```python
from build123d import *

# Parameters (mm, degrees)
CUT_EXTRUDE1_DEPTH  = 3
BOSS_EXTRUDE1_START = 15
SKETCH12_R          = 2
BOSS_EXTRUDE1_DEPTH = 15


with BuildPart() as part:
    # Sketch2 → Revolve1 (revolve)
    with BuildSketch(Plane(origin=(0, 0, 0), x_dir=(0, 0, -1), z_dir=(1, 0, 0))):
        with BuildLine():
            Line((-7, 0), (-7, 3.3))
            Line((-7, 3.3), (-6.8, 3.5))
            Line((-6.8, 3.5), (-3.2, 3.5))
            Line((-3.2, 3.5), (-3, 3.3))
            Line((-3, 3.3), (-3, 2.2))
            ThreePointArc((-3, 2.2), (-2.941421356, 2.058578644), (-2.8, 2))
            Line((-2.8, 2), (6.545336663, 2))
            Line((6.545336663, 2), (7, 1.545336663))
            Line((7, 1.545336663), (7, 0))
            Line((7, 0), (-7, 0))
        make_face()
    revolve(axis=Axis((0, 0, -7), (0, 0, 1)))

    # Sketch3 → Cut-Extrude1 (cut)
    with BuildSketch(Plane.XY.offset(7)):
        Polygon((1.5, -0.866025404), (1.5, 0.866025404), (0, 1.732050808), (-1.5, 0.866025404), (-1.5, -0.866025404), (0, -1.732050808), align=None)
    extrude(amount=-CUT_EXTRUDE1_DEPTH, mode=Mode.SUBTRACT)

    # Cut-Extrude2 cone 1 section (through the dimple's axis) → Cut-Extrude2 (revolve, cut)
    with BuildSketch(Plane(origin=(0, 0, 7), x_dir=(0, -1, 0), z_dir=(1, 0, 0))):
        Polygon((0, 0), (1.875, 0), (0, 1.875), align=None)
    revolve(axis=Axis((0, 0, 7), (0, 0, -1)), mode=Mode.SUBTRACT)

    # Sketch12 → Boss-Extrude1 (add)
    with BuildSketch(Plane(origin=(0, 0, 3), x_dir=(-1, 0, 0), z_dir=(0, 0, -1)).offset(BOSS_EXTRUDE1_START)):
        with Locations(Location((0, 0, 0), (0, 0, 90))):
            Circle(SKETCH12_R)
    extrude(amount=-BOSS_EXTRUDE1_DEPTH)


solid = part.part
```
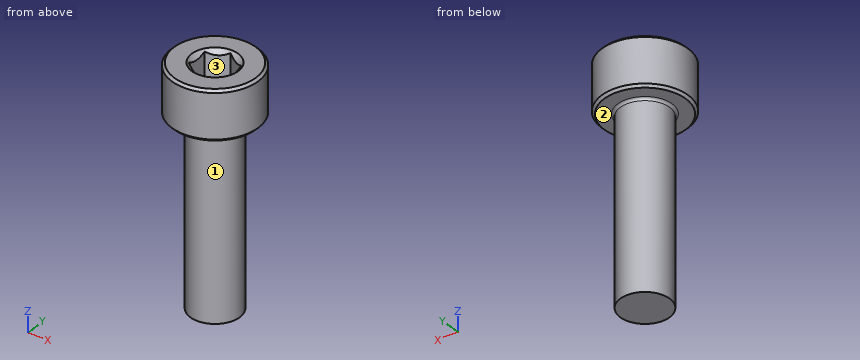
Can you work these out from the model? Positions are in its coordinate system, mm. Face numbers are marked on the shaded views. Give positions to 0.01 mm unless a question says otherwise; leave off trailing zeros. Loops run counter-clockwise (first coordinate to the right, second up) from the corner with the lowest first, then second, coordinate; pieces in that order, holes last. Notation, with made-up numbers: M 0.5,66 L 44.5,66 A29 ccw 44.5,97 Z; hole C 49,-34.75 d5. An arc over 180 degrees is marked long. Use one line per item in the form item = value. Start each with the question number.
(1) I want a section at A-A, the plane z = 5.25. Write out the boundary of the cut face in (x, y).
(2) I want a section at B-B, the plane y = 0. Write out the boundary of the cut face in (x, z) (3 decimals).
(3) Please list where these lines run through material, in increasing order: line 1 (Z direction, x = -2.5, y = 1.25); line 2 (Z direction, x = -0.25, y = -0.25); line 3 (X direction, y = -1.5, z = 6.25).
(4) I want a section at C-C, the plane z = -2.5. Write out the boundary of the cut face in (x, y), and give its area (3 significant figures).
(5) Thinking about a two-plate mould opening in X: for the marked faces 1, 2 and 3, which applies, released by +X, released by -X, zero draft, split by the parting line, or undercut?
(6) I'm going to push flat-ended pins straight in: P1, Ø4, axis at y = 1.5, z = -5, coming from the +X side; P2, Ø1.5, axis at x = 0, y = -0.5, coming from the +Z side; P3, Ø4, axis at x = -2, z = -6, coming from the +Y side. Where does each tip first touch, or does it pass through?
Worked out:
q1.outline = C 0,0 d7; hole M -1.5,-0.87 L 0,-1.73 L 1.5,-0.87 L 1.5,0.87 L 0,1.73 L -1.5,0.87 Z
q2.outline = M -3.5,3.2 L -3.3,3 L -2.2,3 A0.2 cw -2,2.8 L -2,-12 L 2,-12 L 2,2.8 A0.2 cw 2.2,3 L 3.3,3 L 3.5,3.2 L 3.5,6.8 L 3.3,7 L 1.875,7 L 1.5,6.625 L 1.5,4 L -1.5,4 L -1.5,6.625 L -1.875,7 L -3.3,7 L -3.5,6.8 Z
q3.line_1 = 3 to 7
q3.line_2 = -12 to 4
q3.line_3 = -3.16 to -0.4, 0.4 to 3.16
q4.outline = C 0,0 d4
q4.area = 12.6 mm²
q5.face_1 = split by the parting line
q5.face_2 = zero draft
q5.face_3 = undercut
q6.P1 = 2
q6.P2 = 4
q6.P3 = 2
